```python
from build123d import *

# Parameters (mm, degrees)
SM_BASE_FLANGE_1_DEPTH = 5
OTHER_START            = -5
OTHER_1_DEPTH          = 5
SKETCH_8_R             = 5.1
CUT_EXTRUDE_1_DEPTH    = 153.151240547


# Read off the part's stored shape, not the designer's step: Выступы и прорези-Выступ1
# Sheet-metal steps are written as plain solids
with BuildPart() as part:
    # Sketch 1 → Базовая кромка1 (new body)
    with BuildSketch(Plane(origin=(0, 0, 0), x_dir=(1, 0, 0), z_dir=(0, 1, 0))):
        with BuildLine():
            Line((0, -105), (103.662809462, -105))
            Line((103.662809462, -105), (103.662809462, 0))
            Line((103.662809462, 0), (6.25, 0))
            ThreePointArc((6.25, 0), (0, -6.25), (-6.25, 0))
            Line((-6.25, 0), (-105, 0))
            ThreePointArc((-105, 0), (-74.246212025, -74.246212025), (0, -105))
        make_face()
    extrude(amount=-SM_BASE_FLANGE_1_DEPTH)

    # Other 1 outline → Other 1 (add)
    with BuildSketch(Plane(origin=(0, 0, 0), x_dir=(1, 0, 0), z_dir=(0, 1, 0)).offset(OTHER_START)):
        Polygon((98.662809462, -105), (78.662809462, -105), (78.662809462, -108), (80.662809462, -110), (96.662809462, -110), (98.662809462, -108), align=None)
        Polygon((61.831404731, -105), (41.831404731, -105), (41.831404731, -108), (43.831404731, -110), (59.831404731, -110), (61.831404731, -108), align=None)
        Polygon((5, -105), (5, -108), (7, -110), (23, -110), (25, -108), (25, -105), align=None)
    extrude(amount=OTHER_1_DEPTH)

    # Зеркальное отражение1: part across plane


with BuildPart() as part_1:
    add(part.part)
    add(part.part.mirror(Plane(origin=(6.25, -5, 0), x_dir=(1, 0, 0), z_dir=(0, 0, -1))))

    # Эскиз8 → Вырез-Вытянуть1 (cut, through all)
    with BuildSketch(Plane(origin=(0, 0, 0), x_dir=(1, 0, 0), z_dir=(0, 1, 0))):
        with Locations(Location((-65.778483455, 23.941410033, 0), (0, 0, 270))):
            Circle(SKETCH_8_R)
        with Locations(Location((-68.936542711, 12.155372437, 0), (0, 0, 270))):
            Circle(SKETCH_8_R)
        with Locations(Location((-70, 0, 0), (0, 0, 270))):
            Circle(SKETCH_8_R)
        with Locations(Location((-68.936542711, -12.155372437, 0), (0, 0, 270))):
            Circle(SKETCH_8_R)
        with Locations(Location((-65.778483455, -23.941410033, 0), (0, 0, 270))):
            Circle(SKETCH_8_R)
    extrude(amount=-CUT_EXTRUDE_1_DEPTH, mode=Mode.SUBTRACT)


solid = part_1.part
```
CAD build for the part. Positions are in the model's coordinates, mm. A direction names the side the tool comes from. Coordinates: 2 decimals unless noted, no trailing zeros. Order: outer loops, then holes, each group sorted by start corner. A loop starts at its lowest first (then second) coordinate and runs counter-clockwise, first axis right, second up. Notation, with made-up numbers: (45, 70.25) - (76, 70.25) arc R30 cw to (76, 105.25) - close; hole circle Ø7 at (46, 55). An arc over 180 degrees is marked (long way). Use a Markdown table: item, result. Add a question column.
(1) Pull direction X, two halves, no side cores. Call faces 5 (the face through (103.663, -2, -1)), 6 (the face through (15, -3, -110)), 7 (the face through (70, -2, 105)): +X half, -X half, draft (parallel to the pull), parting line (faces both ways), or undercut.
(2) Flat gauge pins, fed straight in: pin 1 (0.9 mm diameter, centred on y = -2, z = 107, fed in from +X); pin 2 (8 mm diameter, centred on x = -70, z = 0, fed in from +Y); pin 3 (1.5 mm diameter, centred on y = -2.5, z = -106.5, fed in from -X); pin 4 (2 mm diameter, centred on x = -8, y = -4, fed in from +Z). Where does each tip first touch, or does it go through?
(3) Which spindle directions (+Z, -Z, +X, -X, +Y, -Y) get a long thin tool onto all of the face, cutting with end or side? Do faces 1 (the face through (70, -2, -105)), 2 (the face through (101, -2, 105)), 3 (the face through (2, -2, -105)), 4 (the face through (33, -2, 105)). Say none if no direction does.
(4) Saw through at A-A (y = -3). Count the separate pieces of the cut face and the enclosed holes in it, then the cut area to 3 significant figures.
(5) Saw through at B-B (x = -86.5). Give the cut face in (y, z), then the cut area to 3 significant figures.
(6) Drill centre lines: line 1 along Z through (x, y) = (62, -4); line 2 along X through (y, z) = (-3.6, -23); line 3 along X through (y, z) = (-1.5, -24.5). Where is each one in solid material? Low to high. Write a range as [from, to].
(7) Saw through at C-C (z = 96). Give the cut face in (x, y), then the cut area to 3 significant figures.
Solved:
| question | item | result |
|---|---|---|
| 1 | face 5 | +X half |
| 1 | face 6 | draft |
| 1 | face 7 | undercut |
| 2 | pin 1 | stops at x = 98.66 |
| 2 | pin 2 | passes through |
| 2 | pin 3 | stops at x = 5 |
| 2 | pin 4 | stops at z = 104.77 |
| 3 | face 1 | -Z, +Y, -Y |
| 3 | face 2 | +Z, +X, +Y, -Y |
| 3 | face 3 | -Z, -X, +Y, -Y |
| 3 | face 4 | +Z, +Y, -Y |
| 4 | separate pieces | 1 |
| 4 | enclosed holes | 6 |
| 4 | area | 39,100 mm² |
| 5 | outline | (-5, -59.52) - (0, -59.52) - (0, 59.52) - (-5, 59.52) - close |
| 5 | area | 595 mm² |
| 6 | line 1 | z = [-105, 105] |
| 6 | line 2 | x = [-102.45, -70.79], [-60.77, 103.66] |
| 6 | line 3 | x = [-102.1, -70.85], [-60.71, 103.66] |
| 7 | outline | (-42.53, -5) - (103.66, -5) - (103.66, 0) - (-42.53, 0) - close |
| 7 | area | 731 mm² |
